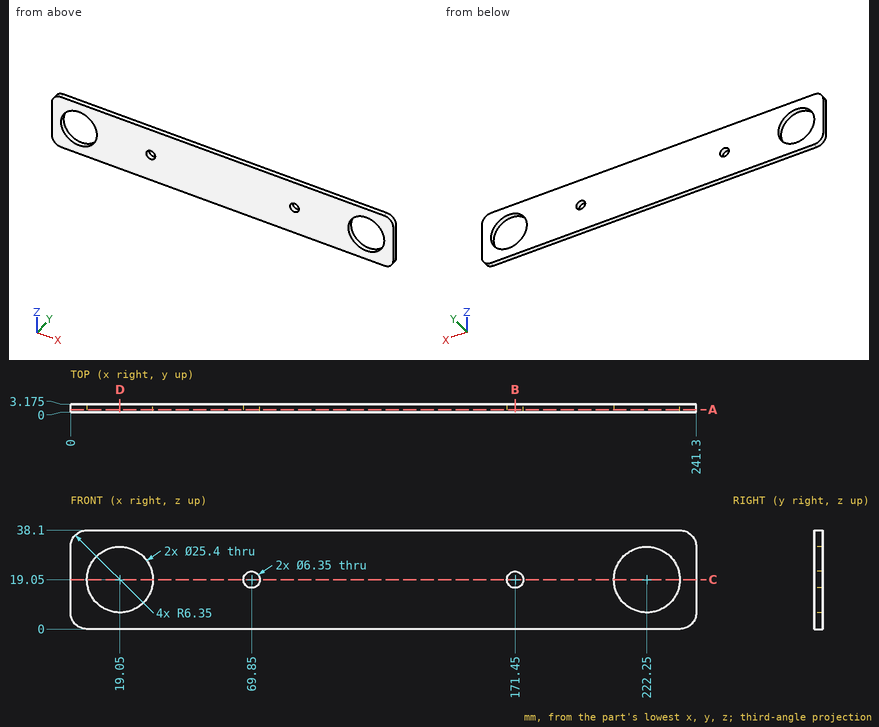
Geometry: see drawing. Coordinates: mm, zero at the bounding-box minimum. Coordinates: 2 decimals unless noted, no trailing zeros. Order: outer loops, then holes, each group sorted by start corner. A loop starts at its lowest first (then second) coordinate and runs counter-clockwise, first axis right, second up. Notation, with made-up numbers: (-12.5, 85.25) -> (35.5, 85.25) arc R22 cw to (35.5, 95.25) -> close; hole circle Ø5 at (-31.75, -40). An arc over 180 degrees is marked (long way). Write each question's results on one line, items separated by ' | '. Start each with the question number.
1) Cut plane D-D, the plane x = 19.05. Output: boundary loops of the cut face in (y, z) (3 decimals).
2) Cut plane C-C, the plane z = 19.05. Output: boundary loops of the cut face in (x, y) (3 decimals), and give its area (3 significant figures).
3) Cut plane B-B, the plane x = 171.45. Output: boundary loops of the cut face in (y, z) (3 decimals), and give its area (3 significant figures).
4) Material intervals for line 1 along X through (y, z) = (0.95, 13.5); line 2 along X through (y, z) = (1.8, 14.5); line 3 along Z through (x, y) = (171.45, 1.6) (3 decimals), sorted ascending.
5) Cut plane A-A, the plane y = 1.05. Output: boundary loops of the cut face in (x, z) (3 decimals).
6) First-contact query: pin 1 (1.5 mm diameter, centred on x = 134.5, z = 5, fed in from -Y). Flat tip, straight axial feed; report the tip coordinate or a pass-through.
Checks:
1) outline: (0, 0) -> (3.175, 0) -> (3.175, 6.35) -> (0, 6.35) -> close; (0, 31.75) -> (3.175, 31.75) -> (3.175, 38.1) -> (0, 38.1) -> close
2) outline: (0, 0) -> (6.35, 0) -> (6.35, 3.175) -> (0, 3.175) -> close; (31.75, 0) -> (66.675, 0) -> (66.675, 3.175) -> (31.75, 3.175) -> close; (73.025, 0) -> (168.275, 0) -> (168.275, 3.175) -> (73.025, 3.175) -> close; (174.625, 0) -> (209.55, 0) -> (209.55, 3.175) -> (174.625, 3.175) -> close; (234.95, 0) -> (241.3, 0) -> (241.3, 3.175) -> (234.95, 3.175) -> close | area: 565 mm^2
3) outline: (0, 0) -> (3.175, 0) -> (3.175, 15.875) -> (0, 15.875) -> close; (0, 22.225) -> (3.175, 22.225) -> (3.175, 38.1) -> (0, 38.1) -> close | area: 101 mm^2
4) line 1: 0 to 7.63, 30.47 to 210.83, 233.67 to 241.3 | line 2: 0 to 7.19, 30.91 to 210.39, 234.11 to 241.3 | line 3: 0 to 15.875, 22.225 to 38.1
5) outline: (0, 6.35) arc R6.35 ccw to (6.35, 0) -> (234.95, 0) arc R6.35 ccw to (241.3, 6.35) -> (241.3, 31.75) arc R6.35 ccw to (234.95, 38.1) -> (6.35, 38.1) arc R6.35 ccw to (0, 31.75) -> close; hole circle Ø25.4 at (19.05, 19.05); hole circle Ø6.35 at (69.85, 19.05); hole circle Ø6.35 at (171.45, 19.05); hole circle Ø25.4 at (222.25, 19.05)
6) pin 1: y = 0
